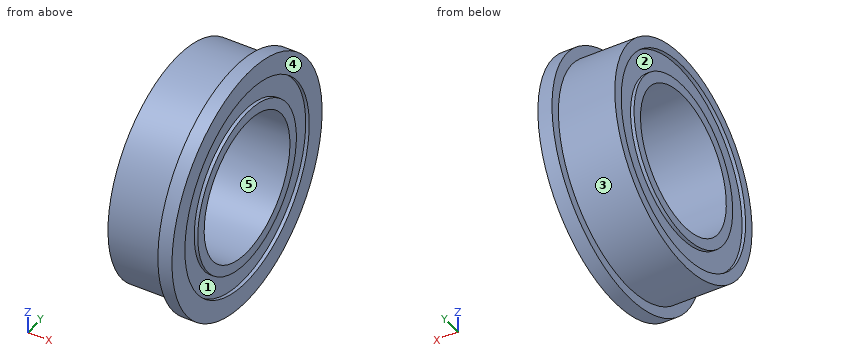
from build123d import *


with BuildPart() as part:
    # 草图1 → 旋转1 (revolve)
    with BuildSketch(Plane(origin=(0, 0, 0), x_dir=(1, 0, 0), z_dir=(0, 1, 0)), mode=Mode.PRIVATE) as revolve_1_sk:
        Polygon((0, 10), (10, 10), (10, 11.5), (9.5, 11.5), (9.5, 14.5), (10, 14.5), (10, 17.5), (8, 17.5), (8, 16), (0, 16), (0, 14.5), (0.5, 14.5), (0.5, 11.5), (0, 11.5), align=None)
    revolve(revolve_1_sk.sketch.rotate(Axis((0, 0, 0), (1, 0, 0)), 180), axis=Axis((0, 0, 0), (1, 0, 0)))


solid = part.part
Can you work these out from the model? Positions are in its coordinate system, mm. Face numbers are marked on the shaded views. A direction names the side the tool comes from. Coordinates: 2 decimals unless noted, no trailing zeros. Order: outer loops, then holes, each group sorted by start corner. A loop starts at its lowest first (then second) coordinate and runs counter-clockwise, first axis right, second up. Notation, with made-up numbers: (75, 1.25) -> (113, 1.25) arc R25 cw to (113, 16.25) -> close; hole circle Ø11 at (76, 39.5). An arc over 180 degrees is marked (long way). Use one line per item in the form item = value.
Q1. Imagine slicing it at A-A, the plane z = 0. List the corners of the cut face in (x, y) for me, then the cut area to 3 significant figures.
From the geometry:
outline = (0, -16) -> (8, -16) -> (8, -17.5) -> (10, -17.5) -> (10, -14.5) -> (9.5, -14.5) -> (9.5, -11.5) -> (10, -11.5) -> (10, -10) -> (0, -10) -> (0, -11.5) -> (0.5, -11.5) -> (0.5, -14.5) -> (0, -14.5) -> close; (0, 10) -> (10, 10) -> (10, 11.5) -> (9.5, 11.5) -> (9.5, 14.5) -> (10, 14.5) -> (10, 17.5) -> (8, 17.5) -> (8, 16) -> (0, 16) -> (0, 14.5) -> (0.5, 14.5) -> (0.5, 11.5) -> (0, 11.5) -> close
area = 120 mm²
Q2. Imagine slicing it at C-C, the plane x = 6.75. List the corners of the cut face in (y, z) for me, then the cut area to 3 significant figures.
From the geometry:
outline = circle Ø32 at (0, 0); hole circle Ø20 at (0, 0)
area = 490 mm²
Q3. Which directions (+Z, -Z, +X, -X, +Y, -Y) give clear straight access to the entire face, cutting with the end or side of a thin tool? Please do the marked faces 1 and 2.
From the geometry:
face_1 = +X
face_2 = -X
Q4. Imagine slicing it at D-D, the plane z = 13.5. List the corners of the cut face in (x, y) for me.
From the geometry:
outline = (0, -8.59) -> (8, -8.59) -> (8, -11.14) -> (10, -11.14) -> (10, -5.29) -> (9.5, -5.29) -> (9.5, 5.29) -> (10, 5.29) -> (10, 11.14) -> (8, 11.14) -> (8, 8.59) -> (0, 8.59) -> (0, 5.29) -> (0.5, 5.29) -> (0.5, -5.29) -> (0, -5.29) -> close
Q5. I need wall thicknesses on L1, parallel to Y at x = 9.85, z = 0; L2, parallel to Y at x = 0.15, z = 0; L3, parallel to Y at x = 7.5, z = 0. Which ranges of each line are inside material? Lowest first, please.
From the geometry:
L1 = -17.5 to -14.5, -11.5 to -10, 10 to 11.5, 14.5 to 17.5
L2 = -16 to -14.5, -11.5 to -10, 10 to 11.5, 14.5 to 16
L3 = -16 to -10, 10 to 16
Q6. We'd pull the mould along Y, two halves only. Please class the marked faces 3, 4 and 5: released by +Y, released by -Y, zero draft, split by the parting line, or undercut.
From the geometry:
face_3 = split by the parting line
face_4 = zero draft
face_5 = undercut
Q7. Will these pins go through, and if not, where does the flat tip stop? P1, Ø5, axis at x = 5, z = 7.5, coming from the -Y side; P2, Ø8.5, axis at y = -0.5, z = -5, coming from the -X side; P3, Ø1, axis at y = 6.5, z = -12, coming from the +X side; P4, Ø2, axis at x = 1.5, z = -13.5, coming from the +Y side.
From the geometry:
P1 = -15.2
P2 = through
P3 = 9.5
P4 = 9.99
